The listing builds one solid part. Answer for the finished solid, in the listing's coordinates (mm). Face numbers are marked on the shaded views. A direction names the side the tool comes from. Round coordinates to 2 decimals unless told otherwise and drop trailing zeros. Order: outer loops, then holes, each group sorted by start corner. A loop starts at its lowest first (then second) coordinate and runs counter-clockwise, first axis right, second up. Notation, with made-up numbers: (88, 68.25) - (116, 68.25) arc R23 ccw to (116, 107.25) - close; hole circle Ø11 at (61.5, 23). An arc over 180 degrees is marked (long way). One line per item, written item: value. Start each with the question number.
1. Section B-B, the plane y = 0 is taken. Give the vertices of the cut face in (x, z) (3 decimals).
2. Straight lines are drawn through the part: line 1 (X direction, y = -9.75, z = 3.25); line 2 (Y direction, x = 10.5, z = 3.5); line 3 (Y direction, x = 0, z = 3.25) (3 decimals). For each, find the intervals that lie inside material, in ascending order.
3. Section C-C, the plane x = 5 is taken. Give the vertices of the cut face in (y, z), then the cut area to 3 significant figures.
4. Section D-D, the plane x = 7.5 is taken. Give the vertices of the cut face in (y, z), then the cut area to 3 significant figures.
5. For a pull along Y with two mould halves and no side action, classify the marked faces 1, 2 and 3 as released by +Y, released by -Y, zero draft, split by the parting line, or undercut.
6. A tool of negligible diameter and unlimited length cuts with its end or side. For the marked faces 4, 5 and 6, from which of +Z, -Z, +X, -X, +Y, -Y can it reach the whole face along a straight path? Write none if from no direction.
7. Flat-ended cylindrical pins translate along their axes: P1, Ø8.5, axis at x = 0, y = 0, coming from the -Z side; P2, Ø1.5, axis at y = -0.5, z = 0.5, coming from the +X side. Find the tip coordinate at first contact, or state that the pin passes through.
8. Section A-A, the plane x = 0 is taken. Give the vertices of the cut face in (y, z) (3 decimals), then the cut area to 3 significant figures.
from build123d import *

# Parameters (mm, degrees)
SKETCH1_R           = 3.675
BOSS_EXTRUDE1_DEPTH = 6.35


with BuildPart() as part:
    # Sketch1 → Boss-Extrude1 (new body)
    with BuildSketch(Plane.XY.offset(6.35)):
        with BuildLine():
            ThreePointArc((-3.880007235, 11.657556143), (-3.94321083, 10.464048215), (-3.841100867, 9.273237808))
            ThreePointArc((-3.841100867, 9.273237808), (-4.169636916, 9.130231284), (-4.492859393, 8.975589663))
            ThreePointArc((-4.492859393, 8.975589663), (-5.325946046, 9.8325742), (-6.269328707, 10.566389588))
            ThreePointArc((-6.269328707, 10.566389588), (-6.642473156, 10.335889983), (-7.007152779, 10.092218849))
            ThreePointArc((-7.007152779, 10.092218849), (-6.731546143, 8.929249868), (-6.298082291, 7.815443351))
            ThreePointArc((-6.298082291, 7.815443351), (-6.573020728, 7.585670296), (-6.839582844, 7.346230451))
            ThreePointArc((-6.839582844, 7.346230451), (-7.880364079, 7.933793461), (-8.992272799, 8.37210256))
            ThreePointArc((-8.992272799, 8.37210256), (-9.285363033, 8.045812868), (-9.566620477, 7.709270006))
            ThreePointArc((-9.566620477, 7.709270006), (-8.974531622, 6.671056802), (-8.244830544, 5.724488154))
            ThreePointArc((-8.244830544, 5.724488154), (-8.443897491, 5.426563413), (-8.632203969, 5.121723338))
            ThreePointArc((-8.632203969, 5.121723338), (-9.79636188, 5.392263959), (-10.986716428, 5.499557573))
            ThreePointArc((-10.986716428, 5.499557573), (-11.176008019, 5.103911846), (-11.351057479, 4.701761955))
            ThreePointArc((-11.351057479, 4.701761955), (-10.490453922, 3.872414387), (-9.523631659, 3.169768972))
            ThreePointArc((-9.523631659, 3.169768972), (-9.630699898, 2.827828636), (-9.725495267, 2.48228466))
            ThreePointArc((-9.725495267, 2.48228466), (-10.918716703, 2.4138853), (-12.091081632, 2.181471139))
            ThreePointArc((-12.091081632, 2.181471139), (-12.161239301, 1.74852224), (-12.215899311, 1.313345113))
            ThreePointArc((-12.215899311, 1.313345113), (-11.156502035, 0.76005199), (-10.030884778, 0.358253958))
            ThreePointArc((-10.030884778, 0.358253958), (-10.037280275, 0), (-10.030884778, -0.358253958))
            ThreePointArc((-10.030884778, -0.358253958), (-11.156502035, -0.76005199), (-12.215899311, -1.313345113))
            ThreePointArc((-12.215899311, -1.313345113), (-12.161239301, -1.74852224), (-12.091081632, -2.181471139))
            ThreePointArc((-12.091081632, -2.181471139), (-10.918716703, -2.4138853), (-9.725495267, -2.48228466))
            ThreePointArc((-9.725495267, -2.48228466), (-9.630699898, -2.827828636), (-9.523631659, -3.169768972))
            ThreePointArc((-9.523631659, -3.169768972), (-10.490453922, -3.872414387), (-11.351057479, -4.701761955))
            ThreePointArc((-11.351057479, -4.701761955), (-11.176008019, -5.103911846), (-10.986716428, -5.499557573))
            ThreePointArc((-10.986716428, -5.499557573), (-9.79636188, -5.392263959), (-8.632203969, -5.121723338))
            ThreePointArc((-8.632203969, -5.121723338), (-8.443897491, -5.426563413), (-8.244830544, -5.724488154))
            ThreePointArc((-8.244830544, -5.724488154), (-8.974531622, -6.671056802), (-9.566620477, -7.709270006))
            ThreePointArc((-9.566620477, -7.709270006), (-9.285363033, -8.045812868), (-8.992272799, -8.37210256))
            ThreePointArc((-8.992272799, -8.37210256), (-7.880364079, -7.933793461), (-6.839582844, -7.346230451))
            ThreePointArc((-6.839582844, -7.346230451), (-6.573020728, -7.585670296), (-6.298082291, -7.815443351))
            ThreePointArc((-6.298082291, -7.815443351), (-6.731546143, -8.929249868), (-7.007152779, -10.092218849))
            ThreePointArc((-7.007152779, -10.092218849), (-6.642473156, -10.335889983), (-6.269328707, -10.566389588))
            ThreePointArc((-6.269328707, -10.566389588), (-5.325946046, -9.8325742), (-4.492859393, -8.975589663))
            ThreePointArc((-4.492859393, -8.975589663), (-4.169636916, -9.130231284), (-3.841100867, -9.273237808))
            ThreePointArc((-3.841100867, -9.273237808), (-3.94321083, -10.464048215), (-3.880007235, -11.657556143))
            ThreePointArc((-3.880007235, -11.657556143), (-3.461449609, -11.788614761), (-3.038480888, -11.904650573))
            ThreePointArc((-3.038480888, -11.904650573), (-2.340051539, -10.934778255), (-1.782151195, -9.87779998))
            ThreePointArc((-1.782151195, -9.87779998), (-1.428453919, -9.935115234), (-1.072936295, -9.979769688))
            ThreePointArc((-1.072936295, -9.979769688), (-0.835420026, -11.151111607), (-0.438526581, -12.278467567))
            ThreePointArc((-0.438526581, -12.278467567), (0, -12.28629608), (0.438526581, -12.278467567))
            ThreePointArc((0.438526581, -12.278467567), (0.835420026, -11.151111607), (1.072936295, -9.979769688))
            ThreePointArc((1.072936295, -9.979769688), (1.428453919, -9.935115234), (1.782151195, -9.87779998))
            ThreePointArc((1.782151195, -9.87779998), (2.340051539, -10.934778255), (3.038480888, -11.904650573))
            ThreePointArc((3.038480888, -11.904650573), (3.461449609, -11.788614761), (3.880007235, -11.657556143))
            ThreePointArc((3.880007235, -11.657556143), (3.94321083, -10.464048215), (3.841100867, -9.273237808))
            ThreePointArc((3.841100867, -9.273237808), (4.169636916, -9.130231284), (4.492859393, -8.975589663))
            ThreePointArc((4.492859393, -8.975589663), (5.325946046, -9.8325742), (6.269328707, -10.566389588))
            ThreePointArc((6.269328707, -10.566389588), (6.642473156, -10.335889983), (7.007152779, -10.092218849))
            ThreePointArc((7.007152779, -10.092218849), (6.731546143, -8.929249868), (6.298082291, -7.815443351))
            ThreePointArc((6.298082291, -7.815443351), (6.573020728, -7.585670296), (6.839582844, -7.346230451))
            ThreePointArc((6.839582844, -7.346230451), (7.880364079, -7.933793461), (8.992272799, -8.37210256))
            ThreePointArc((8.992272799, -8.37210256), (9.285363033, -8.045812868), (9.566620477, -7.709270006))
            ThreePointArc((9.566620477, -7.709270006), (8.974531622, -6.671056802), (8.244830544, -5.724488154))
            ThreePointArc((8.244830544, -5.724488154), (8.443897491, -5.426563413), (8.632203969, -5.121723338))
            ThreePointArc((8.632203969, -5.121723338), (9.79636188, -5.392263959), (10.986716428, -5.499557573))
            ThreePointArc((10.986716428, -5.499557573), (11.176008019, -5.103911846), (11.351057479, -4.701761955))
            ThreePointArc((11.351057479, -4.701761955), (10.490453922, -3.872414387), (9.523631659, -3.169768972))
            ThreePointArc((9.523631659, -3.169768972), (9.630699898, -2.827828636), (9.725495267, -2.48228466))
            ThreePointArc((9.725495267, -2.48228466), (10.918716703, -2.4138853), (12.091081632, -2.181471139))
            ThreePointArc((12.091081632, -2.181471139), (12.161239301, -1.74852224), (12.215899311, -1.313345113))
            ThreePointArc((12.215899311, -1.313345113), (11.156502035, -0.76005199), (10.030884778, -0.358253958))
            ThreePointArc((10.030884778, -0.358253958), (10.037280275, 0), (10.030884778, 0.358253958))
            ThreePointArc((10.030884778, 0.358253958), (11.156502035, 0.76005199), (12.215899311, 1.313345113))
            ThreePointArc((12.215899311, 1.313345113), (12.161239301, 1.74852224), (12.091081632, 2.181471139))
            ThreePointArc((12.091081632, 2.181471139), (10.918716703, 2.4138853), (9.725495267, 2.48228466))
            ThreePointArc((9.725495267, 2.48228466), (9.630699898, 2.827828636), (9.523631659, 3.169768972))
            ThreePointArc((9.523631659, 3.169768972), (10.490453922, 3.872414387), (11.351057479, 4.701761955))
            ThreePointArc((11.351057479, 4.701761955), (11.176008019, 5.103911846), (10.986716428, 5.499557573))
            ThreePointArc((10.986716428, 5.499557573), (9.79636188, 5.392263959), (8.632203969, 5.121723338))
            ThreePointArc((8.632203969, 5.121723338), (8.443897491, 5.426563413), (8.244830544, 5.724488154))
            ThreePointArc((8.244830544, 5.724488154), (8.974531622, 6.671056802), (9.566620477, 7.709270006))
            ThreePointArc((9.566620477, 7.709270006), (9.285363033, 8.045812868), (8.992272799, 8.37210256))
            ThreePointArc((8.992272799, 8.37210256), (7.880364079, 7.933793461), (6.839582844, 7.346230451))
            ThreePointArc((6.839582844, 7.346230451), (6.573020728, 7.585670296), (6.298082291, 7.815443351))
            ThreePointArc((6.298082291, 7.815443351), (6.731546143, 8.929249868), (7.007152779, 10.092218849))
            ThreePointArc((7.007152779, 10.092218849), (6.642473156, 10.335889983), (6.269328707, 10.566389588))
            ThreePointArc((6.269328707, 10.566389588), (5.325946046, 9.8325742), (4.492859393, 8.975589663))
            ThreePointArc((4.492859393, 8.975589663), (4.169636916, 9.130231284), (3.841100867, 9.273237808))
            ThreePointArc((3.841100867, 9.273237808), (3.94321083, 10.464048215), (3.880007235, 11.657556143))
            ThreePointArc((3.880007235, 11.657556143), (3.461449609, 11.788614761), (3.038480888, 11.904650573))
            ThreePointArc((3.038480888, 11.904650573), (2.340051539, 10.934778255), (1.782151195, 9.87779998))
            ThreePointArc((1.782151195, 9.87779998), (1.428453919, 9.935115234), (1.072936295, 9.979769688))
            ThreePointArc((1.072936295, 9.979769688), (0.835420026, 11.151111607), (0.438526581, 12.278467567))
            ThreePointArc((0.438526581, 12.278467567), (0, 12.28629608), (-0.438526581, 12.278467567))
            ThreePointArc((-0.438526581, 12.278467567), (-0.835420026, 11.151111607), (-1.072936295, 9.979769688))
            ThreePointArc((-1.072936295, 9.979769688), (-1.428453919, 9.935115234), (-1.782151195, 9.87779998))
            ThreePointArc((-1.782151195, 9.87779998), (-2.340051539, 10.934778255), (-3.038480888, 11.904650573))
            ThreePointArc((-3.038480888, 11.904650573), (-3.461449609, 11.788614761), (-3.880007235, 11.657556143))
        make_face()
        Circle(SKETCH1_R, mode=Mode.SUBTRACT)
    extrude(amount=-BOSS_EXTRUDE1_DEPTH)


solid = part.part
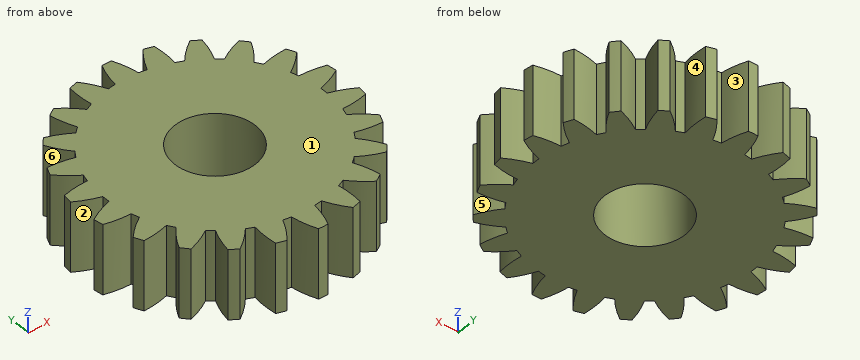
Answer list:
1. outline: (-10.037, 0) - (-3.675, 0) - (-3.675, 6.35) - (-10.037, 6.35) - close; (3.675, 0) - (10.037, 0) - (10.037, 6.35) - (3.675, 6.35) - close
2. line 1: x = -6.94 to -5.24, -3.9 to 3.9, 5.24 to 6.94
2. line 2: y = -5.48 to -3.88, -2.46 to -0.5, 0.5 to 2.46, 3.88 to 5.48
2. line 3: y = -12.286 to -3.675, 3.675 to 12.286
3. outline: (-9.53, 0) - (9.53, 0) - (9.53, 6.35) - (-9.53, 6.35) - close
3. area: 121 mm²
4. outline: (-7.74, 0) - (7.74, 0) - (7.74, 6.35) - (-7.74, 6.35) - close
4. area: 98.3 mm²
5. face 1: zero draft
5. face 2: undercut
5. face 3: released by +Y
6. face 4: +Z, -Z
6. face 5: +Z, -Z, +X
6. face 6: +Z, -Z, -X
7. P1: stops at z = 0
7. P2: stops at x = 12.11
8. outline: (-12.286, 0) - (-3.675, 0) - (-3.675, 6.35) - (-12.286, 6.35) - close; (3.675, 0) - (12.286, 0) - (12.286, 6.35) - (3.675, 6.35) - close
8. area: 109 mm²
